```python
from build123d import *

# Parameters (mm, degrees)
F0_W            = 60
F0_H            = 100
F1_DEPTH        = 10
F2_W            = 12
F2_H            = 100
F3_DEPTH        = 40
F5_W            = 60
F5_H            = 100
F6_DEPTH        = 12
F7_W            = 12
F7_H            = 100
F8_DEPTH        = 40
F10_D           = 5
F10_CSINK_D     = 12
F10_CSINK_ANGLE = 90
F12_D           = 5
F13_R           = 8
F14_DEPTH       = 3
F16_D           = 6.5
F18_D           = 6.5
F20_D           = 5.5
F22_D           = 15.5


with BuildPart() as f1:
    # F0 (on Front) → F1 (new body)
    with BuildSketch(Plane.XZ):
        Rectangle(F0_W, F0_H)
    extrude(amount=F1_DEPTH)

    # F2 (on face) → F3 (join)
    with BuildSketch(Plane.XZ.offset(10)):
        with Locations((-24, 0)):
            Rectangle(F2_W, F2_H)
    extrude(amount=F3_DEPTH)


with BuildPart() as f6:
    # F5 (on Front) → F6 (new body)
    with BuildSketch(Plane.XZ):
        Rectangle(F5_W, F5_H)
    extrude(amount=F6_DEPTH)

    # F7 (on face) → F8 (join)
    with BuildSketch(Plane(origin=(0, 0, 0), x_dir=(-1, 0, 0), z_dir=(0, 1, 0))):
        with Locations((24, 0)):
            Rectangle(F7_W, F7_H)
    extrude(amount=F8_DEPTH)

    # F10 (through all)
    with Locations(Plane.XZ.offset(12)):
        with Locations((-2, -8.5), (-2, -20.5)):
            CounterSinkHole(F10_D / 2, F10_CSINK_D / 2, counter_sink_angle=F10_CSINK_ANGLE)

    # F12 (through all)
    with Locations(Plane.XZ.offset(12)):
        with Locations((15.5, -8.5), (15.5, -20.5)):
            Hole(F12_D / 2)

    # F13 (on face) → F14 (cut)
    with BuildSketch(Plane.YZ.offset(-18)):
        with Locations((20, 6)):
            Circle(F13_R)
        with Locations((20, -34)):
            Circle(F13_R)
    extrude(amount=-F14_DEPTH, mode=Mode.SUBTRACT)

    # F16 (through all)
    with Locations(Plane.YZ.offset(-21)):
        with Locations((20, 6)):
            Hole(F16_D / 2)

    # F18 (through all)
    with Locations(Plane.YZ.offset(-21)):
        with Locations((20, -34)):
            Hole(F18_D / 2)

    # F20 (through all)
    with Locations(Plane.YZ.offset(-18)):
        with Locations((20, 41)):
            Hole(F20_D / 2)

    # F22 (through all)
    with Locations(Plane.YZ.offset(-18)):
        with Locations((20, -14)):
            Hole(F22_D / 2)


solid = f6.part
```
Could you check a few things on this model? Use its own coordinates, in mm. A direction names the side the tool comes from. Coordinates: 2 decimals unless noted, no trailing zeros. Write each loop counter-clockwise with the first axis right and the second up, starting at its lowest first coordinate (ties: lowest second). Pieces come first, ordered by that corner, then holes. Notation, with made-up numbers: (42, 29) -> (70, 29) arc R25 cw to (70, 50) -> close; hole circle Ø10 at (34.5, 10.25). An arc over 180 degrees is marked (long way). Write item = value, one per line. Start each with the question number.
(1) I need wall thicknesses on line 1 (Z direction, x = -2, y = -5); line 2 (Z direction, x = -25.25, y = 20); line 3 (X direction, y = -3, z = -8). Which ranges of each line are inside material? Lowest first, please. Write a range as [from, to].
(2) I want a section at B-B (y = 20). Please give me the cut outline in (x, z).
(3) I want a section at D-D (z = 6). Please give me the cut outline in (x, y), plus the area to 3 significant figures.
(4) We'd pull the mould along Y, two halves only. Please class faces 4 (the face through (17.5, -5.9, -10)), 5 (the face through (-24.084, 20.358, 43.727)), 6 (the face through (-25.563, 23.247, 6.143)), 7 (the face through (-1.421, -8.67, -23.106)): released by +Y, released by -Y, zero draft, split by the parting line, or undercut.
(5) Which directions (+Z, -Z, +X, -X, +Y, -Y) give clear straight access to the entire face, cutting with the end or side of a thin tool? Please do faces 1 (the face through (0, -12, 1)), 2 (the face through (-21, 19.9, 2.6)), 3 (the face through (-18, 15, -1)).
(6) I want a section at A-A (z = 41). Please give me the cut outline in (x, y).
(7) I want a section at C-C (z = -8.5). Please give me the cut outline in (x, y), plus the area to 3 significant figures.
(8) Will these pins go through, and if not, where does the flat tip stop? pin 1 (12.5 mm diameter, centred on y = 20, z = -14, fed in from -X); pin 2 (21 mm diameter, centred on y = 20, z = 6, fed in from +X); pin 3 (5 mm diameter, centred on y = 17.5, z = -31, fed in from +X); pin 4 (8 mm diameter, centred on x = 17, z = 26.5, fed in from +Y).
Result set:
q1.line_1 = [-50, -23], [-18, -11], [-6, 50]
q1.line_2 = [-50, -37.25], [-30.75, -21.75], [-6.25, 2.75], [9.25, 38.25], [43.75, 50]
q1.line_3 = [-30, -4.45], [0.45, 13.05], [17.95, 30]
q2.outline = (-30, -50) -> (-18, -50) -> (-18, -42) -> (-21, -42) -> (-21, -37.25) -> (-30, -37.25) -> close; (-30, -30.75) -> (-21, -30.75) -> (-21, -26) -> (-18, -26) -> (-18, -21.75) -> (-30, -21.75) -> close; (-30, -6.25) -> (-18, -6.25) -> (-18, -2) -> (-21, -2) -> (-21, 2.75) -> (-30, 2.75) -> close; (-30, 9.25) -> (-21, 9.25) -> (-21, 14) -> (-18, 14) -> (-18, 38.25) -> (-30, 38.25) -> close; (-30, 43.75) -> (-18, 43.75) -> (-18, 50) -> (-30, 50) -> close
q3.outline = (-30, -12) -> (30, -12) -> (30, 0) -> (-18, 0) -> (-18, 12) -> (-21, 12) -> (-21, 16.75) -> (-30, 16.75) -> close; (-30, 23.25) -> (-21, 23.25) -> (-21, 28) -> (-18, 28) -> (-18, 40) -> (-30, 40) -> close
q3.area = 1,090 mm2
q4.face_4 = zero draft
q4.face_5 = undercut
q4.face_6 = undercut
q4.face_7 = released by -Y
q5.face_1 = +Z, -Z, +X, -X, -Y
q5.face_2 = +X
q5.face_3 = +Z, -Z, +X, +Y
q6.outline = (-30, -12) -> (30, -12) -> (30, 0) -> (-18, 0) -> (-18, 17.25) -> (-30, 17.25) -> close; (-30, 22.75) -> (-18, 22.75) -> (-18, 40) -> (-30, 40) -> close
q7.outline = (-30, -12) -> (-8, -12) -> (-4.5, -8.5) -> (-4.5, 0) -> (-18, 0) -> (-18, 14.54) -> (-30, 14.54) -> close; (-30, 25.46) -> (-18, 25.46) -> (-18, 40) -> (-30, 40) -> close; (0.5, -8.5) -> (4, -12) -> (13, -12) -> (13, 0) -> (0.5, 0) -> close; (18, -12) -> (30, -12) -> (30, 0) -> (18, 0) -> close
q7.area = 937 mm2
q8.pin_1 = through
q8.pin_2 = -18
q8.pin_3 = -21
q8.pin_4 = 0
